Check sheet for the modelled part. Datum: model origin and axes. Units: mm. Give positions to 0.01 mm unless a question says otherwise; leave off trailing zeros. Write each loop counter-clockwise with the first axis right and the second up, starting at its lowest first coordinate (ties: lowest second). Pieces come first, ordered by that corner, then holes. Notation, with made-up numbers: (14.5, 22.5) -> (68.5, 22.5) arc R5 cw to (68.5, 27.5) -> close; hole circle Ø11 at (68, -6.75). An arc over 180 degrees is marked (long way). Return JSON: item names as keys, results as strings.
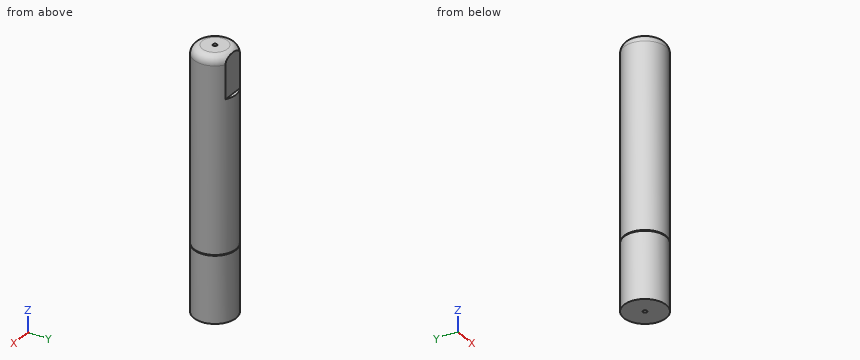
from build123d import *

# Parameters (mm, degrees)
SKETCH3_R          = 0.25
CUT_EXTRUDE1_DEPTH = 50
FILLET1_R          = 1
CUT_EXTRUDE2_START = -5
CUT_EXTRUDE2_DEPTH = 5


with BuildPart() as part:
    # Sketch1 → Revolve1 (revolve)
    with BuildSketch(Plane(origin=(0, 0, 0), x_dir=(0, 0, -1), z_dir=(1, 0, 0)), mode=Mode.PRIVATE) as revolve1_sk:
        Polygon((24.740167046, 48.133333333), (47.640167046, 48.133333333), (47.640167046, 47.633333333), (47.740167046, 47.633333333), (47.740167046, 48.133333333), (50.640167046, 48.133333333), (52.640167046, 48.133333333), (55.640167046, 48.133333333), (55.640167046, 45.633333333), (24.740167046, 45.633333333), align=None)
    revolve(revolve1_sk.sketch.rotate(Axis((0, 45.633333333, -15.940167046), (0, 0, -1)), 90), axis=Axis((0, 45.633333333, -15.940167046), (0, 0, -1)))

    # Sketch3 → Cut-Extrude1 (cut)
    with BuildSketch(Plane.XY.offset(-24.740167046)):
        with Locations((0, 45.633333333)):
            Circle(SKETCH3_R)
    extrude(amount=-CUT_EXTRUDE1_DEPTH, mode=Mode.SUBTRACT)

    # Fillet1
    fillet1_edges = [part.edges().sort_by_distance(p)[0] for p in [
        (-2.5, 45.633333333, -24.740167046),
    ]]
    fillet(fillet1_edges, radius=FILLET1_R)

    # Sketch2 → Cut-Extrude2 (cut)
    with BuildSketch(Plane.XY.offset(-24.740167046).offset(CUT_EXTRUDE2_START)):
        with BuildLine():
            Line((-1.328346703, 47.751232065), (1.328346703, 47.751232065))
            ThreePointArc((1.328346703, 47.751232065), (0.691105336, 48.035909745), (0, 48.133333333))
            ThreePointArc((0, 48.133333333), (-0.691105336, 48.035909745), (-1.328346703, 47.751232065))
        make_face()
    extrude(amount=CUT_EXTRUDE2_DEPTH, mode=Mode.SUBTRACT)


solid = part.part
(1) Depth check by flat-ended pin: pin 1 Ø1.3 at (x, z) = (-0.5, -27) entering from +Y; pin 2 Ø1.5 at (x, z) = (-1.5, -36.5) entering from -Y; pin 3 Ø2 at (y, z) = (47.5, -52) entering from -X (3 decimals). Enter the tip coordinate at first touch or a pass-through.
Reply:
{"pin 1": "y = 47.75", "pin 2": "y = 43.25", "pin 3": "x = -2.345"}
(2) Cross-section at A-A on z = -32. Enter the section's corners in (x, y), then the cut area to 3 significant figures.
Reply:
{"outline": "circle Ø5 at (0, 45.63); hole circle Ø0.5 at (0, 45.63)", "area": "19.4 mm^2"}
(3) Thickness scan on L1, parallel to Y at x = 0, z = -41.5; L2, parallel to Z at x = 0, y = 43.8; L3, parallel to Y at x = -2.05, z = -53. Record the ranges inside material, lowest first.
Reply:
{"L1": "43.13 to 45.38, 45.88 to 48.13", "L2": "-55.64 to -24.8", "L3": "44.2 to 47.06"}
